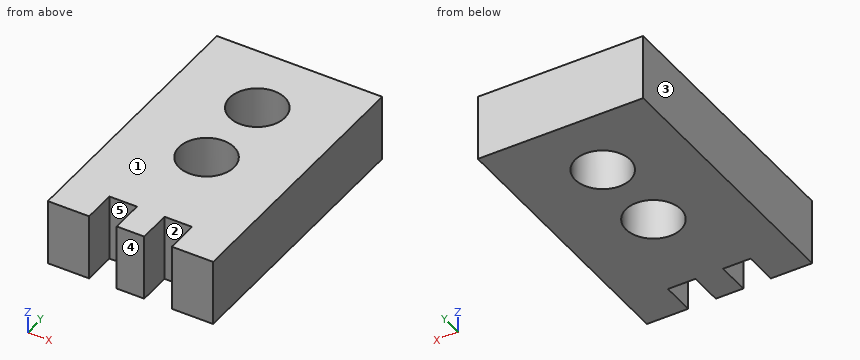
from build123d import *

# Parameters (mm, degrees)
F1_DEPTH = 12
F2_R     = 5
F3_DEPTH = 77.7


with BuildPart() as f1:
    # F0 (on Top) → F1 (new body)
    with BuildSketch(Plane.XY):
        Polygon((-20.183631, 5.870848), (-50.183631, 5.870848), (-50.183631, -44.129152), (-42.683631, -44.129152), (-42.683631, -38.129152), (-37.683631, -38.129152), (-37.683631, -44.129152), (-32.683631, -44.129152), (-32.683631, -38.129152), (-27.683631, -38.129152), (-27.683631, -44.129152), (-20.183631, -44.129152), align=None)
    extrude(amount=F1_DEPTH)

    # F2 (on Top) → F3 (cut)
    with BuildSketch(Plane.XY):
        with Locations((-35.183631, -6.629152)):
            Circle(F2_R)
        with Locations((-35.183631, -21.629152)):
            Circle(F2_R)
    extrude(amount=F3_DEPTH, mode=Mode.SUBTRACT)


solid = f1.part
Geometry check sheet. Reference: the model listing, model coordinates, mm. Face numbers are marked on the shaded views. A direction names the side the tool comes from. Give positions to 0.01 mm unless a question says otherwise; leave off trailing zeros. Loops run counter-clockwise (first coordinate to the right, second up) from the corner with the lowest first, then second, coordinate; pieces in that order, holes last. Notation, with made-up numbers: (13, 50.5) -> (60, 50.5) arc R24 cw to (60, 87.5) -> close; hole circle Ø5 at (13, 67). An arc over 180 degrees is marked (long way). Answer in a Markdown table with one row per item. Add a question column.
1) Draft check along X on the marked faces 1, 2 and 3. Enter one of: pulls with the +X half, pulls with the -X half, needs draft (parallel to the pull), parting line crosses it, or undercut.
2) Gauge pin test, flat ends, axial feed: P1, Ø4, axis at x = -30.5, z = 6.5, coming from the -Y side; P2, Ø10, axis at x = -37.5, y = -25, coming from the -Z side. Record the tip position at first contact, or that the pin passes through.
3) Material ranges on probe 1 along Y at (x, z) = (-38.5, 7.5); probe 2 along Y at (x, z) = (-30.75, 10); probe 3 along X at (y, z) = (-9.5, 10.5), recorded low to high. Write a range as from..to.
4) Cross-section at D-D on x = -30.75. Record the boundary of the cut face in (y, z).
5) Cross-section at A-A on y = -39.5. Record the boundary of the cut face in (x, z).
6) Cross-section at C-C on z = 3.5. Record the boundary of the cut face in (x, y).
7) Set-up check for the marked faces 4 and 5: record each of +Z, -Z, +X, -X, +Y, -Y from which the full face is reachable in a straight line by a thin tool's end or side.
8) Cross-section at B-B on y = -5. Record the boundary of the cut face in (x, z), and give its area (3 significant figures).
Outcome:
| question | item | result |
|---|---|---|
| 1 | face 1 | needs draft |
| 1 | face 2 | undercut |
| 1 | face 3 | pulls with the -X half |
| 2 | P1 | stops at y = -38.13 |
| 2 | P2 | stops at z = 0 |
| 3 | probe 1 | y = -38.13..-25.37, -17.89..-10.37, -2.89..5.87 |
| 3 | probe 2 | y = -38.13..-23.94, -19.32..-8.94, -4.32..5.87 |
| 3 | probe 3 | x = -50.18..-39.28, -31.09..-20.18 |
| 4 | outline | (-38.13, 0) -> (-23.94, 0) -> (-23.94, 12) -> (-38.13, 12) -> close; (-19.32, 0) -> (-8.94, 0) -> (-8.94, 12) -> (-19.32, 12) -> close; (-4.32, 0) -> (5.87, 0) -> (5.87, 12) -> (-4.32, 12) -> close |
| 5 | outline | (-50.18, 0) -> (-42.68, 0) -> (-42.68, 12) -> (-50.18, 12) -> close; (-37.68, 0) -> (-32.68, 0) -> (-32.68, 12) -> (-37.68, 12) -> close; (-27.68, 0) -> (-20.18, 0) -> (-20.18, 12) -> (-27.68, 12) -> close |
| 6 | outline | (-50.18, -44.13) -> (-42.68, -44.13) -> (-42.68, -38.13) -> (-37.68, -38.13) -> (-37.68, -44.13) -> (-32.68, -44.13) -> (-32.68, -38.13) -> (-27.68, -38.13) -> (-27.68, -44.13) -> (-20.18, -44.13) -> (-20.18, 5.87) -> (-50.18, 5.87) -> close; hole circle Ø10 at (-35.18, -21.63); hole circle Ø10 at (-35.18, -6.63) |
| 7 | face 4 | +Z, -Z, +X, -X, -Y |
| 7 | face 5 | +Z, -Z, -Y |
| 8 | outline | (-50.18, 0) -> (-39.91, 0) -> (-39.91, 12) -> (-50.18, 12) -> close; (-30.46, 0) -> (-20.18, 0) -> (-20.18, 12) -> (-30.46, 12) -> close |
| 8 | area | 247 mm^2 |
